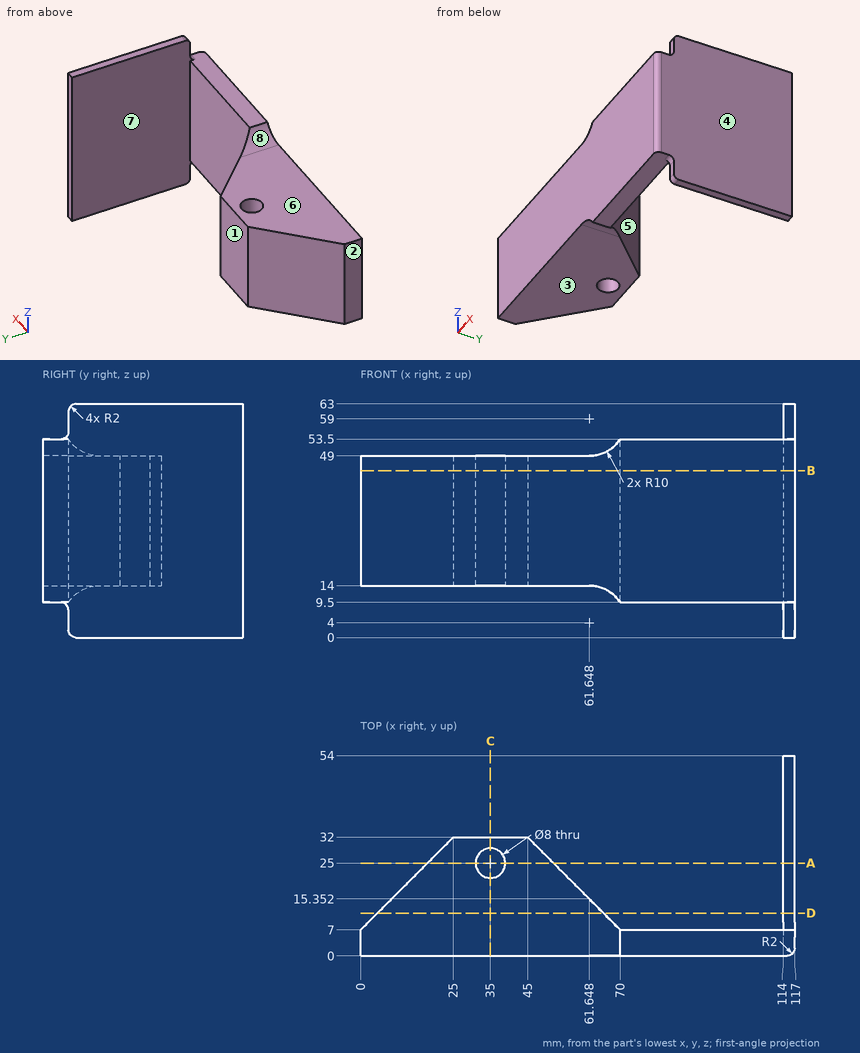
Could you check a few things on this drawing? It's one solid part, dimensions in mm from its lowest x, y, z. A direction names the side the tool comes from. Round coordinates to 2 decimals unless told otherwise and drop trailing zeros. Order: outer loops, then holes, each group sorted by start corner. A loop starts at its lowest first (then second) coordinate and runs counter-clockwise, first axis right, second up. Notation, with made-up numbers: M -30,0.5 L 29,0.5 A20 cw 29,37.5 Z; hole C -26.5,-20 d3. An arc over 180 degrees is marked long. Return JSON: item names as keys, results as strings. Group by question number.
1. If we section it at C-C on x = 35: List the corners of the cut face in (y, z) for me, then the cut area to 3 significant figures.
2. If we mould it in two halves opening along X, with no side actions, what happens to the marked faces 6, 7 and 8? For each: pulls with the +X half, pulls with the -X half, needs draft (parallel to the pull), parting line crosses it, or undercut.
3. On a 3-axis mill with a long thin cutter (end or side, diameter ignored), from which of +Z, -Z, +X, -X, +Y, -Y can I reach the whole of each face in a straight line? I mean the marked faces 1, 2, 3, 4 and 5. Say none if no direction works.
4. If we section it at D-D on y = 11.5: List the corners of the cut face in (x, z) for me.
5. I'm going to push flat-ended pins straight in: pin 1 Ø4 at (x, z) = (39.5, 23.5) entering from +Y; pin 2 Ø1 at (x, z) = (20, 42.5) entering from +Y; pin 3 Ø16 at (x, y) = (32, 11.5) entering from +Z; pin 4 Ø5 at (x, y) = (35, 25) entering from -Z. Where does each tip first touch, or does it pass through?
6. If we section it at A-A on y = 25: List the corners of the cut face in (x, z) for me, then the cut area to 3 significant figures.
7. If we section it at B-B on z = 45: List the corners of the cut face in (x, y) for me, then the cut area to 3 significant figures.
8. Please list where these lines run through material, in increasing order: probe 1 along Y at (x, z) = (35, 26.5); probe 2 along X at (y, z) = (22, 38) (1 decimal); probe 3 along Y at (x, z) = (90, 13).
Reply:
{
 "1": {"outline": "M 0,14 L 21,14 L 21,49 L 0,49 Z; M 29,14 L 32,14 L 32,49 L 29,49 Z", "area": "840 mm^2"},
 "2": {"face 6": "needs draft", "face 7": "undercut", "face 8": "pulls with the -X half"},
 "3": {"face 1": "+Z, -Z, -X, +Y", "face 2": "+Z, -Z, -X, +Y, -Y", "face 3": "-Z, -X, +Y, -Y", "face 4": "+Z, -Z, +X, +Y, -Y", "face 5": "+Z, -Z, +Y"},
 "4": {"outline": "M 4.5,14 L 61.65,14 A10 cw 65.5,13.23 L 65.5,49.77 A10 cw 61.65,49 L 4.5,49 Z; M 114,0 L 117,0 L 117,63 L 114,63 Z"},
 "5": {"pin 1": "y = 32", "pin 2": "y = 27.5", "pin 3": "z = 49", "pin 4": "through"},
 "6": {"outline": "M 18,14 L 31,14 L 31,49 L 18,49 Z; M 39,14 L 52,14 L 52,49 L 39,49 Z; M 114,0 L 117,0 L 117,63 L 114,63 Z", "area": "1,100 mm^2"},
 "7": {"outline": "M 0,0 L 115,0 A2 ccw 117,2 L 117,54 L 114,54 L 114,7 L 70,7 L 45,32 L 25,32 L 0,7 Z; hole C 35,25 d8", "area": "2,030 mm^2"},
 "8": {"probe 1": "0 to 21, 29 to 32", "probe 2": "15 to 32.4, 37.6 to 55, 114 to 117", "probe 3": "0 to 7"}
}
